Autodesk Inventor part; units mm, degrees
ref_plane "YZ Plane" through (0, 0, 0) normal (1, 0, 0) x (0, 1, 0)
ref_plane "XZ Plane" through (0, 0, 0) normal (0, 1, 0) x (-1, 0, 0)
ref_plane "XY Plane" through (0, 0, 0) normal (0, 0, 1) x (1, 0, 0)
sketch "Sketch1" plane through (0, 0, 0) normal (0, 1, 0) x (-1, 0, 0)
  line L0 (50, 0) -> (50, 40)
  line L1 (50, 40) -> (0, 40)
  line L2 (0, 40) -> (0, 0)
  line L3 (0, 0) -> (10, 0)
  line L4 (10, 0) -> (10, 10)
  line L5 (10, 10) -> (10, 30)
  circle A0 centre (10, 30) radius 3.1
  circle A1 centre (10, 10) radius 3.1
  line L6 (45.5, 0) -> (45.5, 11.4783)
  line L7 (0, 0) -> (33.5, 0)
  line L8 (35.5, 0) -> (35.5, 18.6699)
  line L9 (50, 40) -> (45.5, 40)
  line L10 (45.5, 40) -> (45.5, 35.5)
  line L11 (45.5, 35.5) -> (45.5, 34.5217)
  line L12 (45.5, 23) -> (33, 23)
  arc A2 (45.5, 11.4783) -> (33, 40) centre (33, 23) ccw
  line L13 (0, 0) -> (33.5, 0)
  line L14 (35.5, 0) -> (45.5, 0)
  line L15 (33.5, 0) -> (33.5, 18.0251)
  line L16 (0, 0) -> (33.5, 0)
  line L17 (35.5, 0) -> (45.5, 0)
  line L18 (33, 23) -> (28, 23)
  line L19 (33, 23) -> (38, 23)
  arc A3 (35.5, 18.6699) -> (38, 23) centre (33, 23) ccw
  arc A4 (28, 23) -> (33.5, 18.0251) centre (33, 23) ccw
  dimension "d0" = 50
  dimension "d1" = 40
  dimension "d2" = 10
  dimension "d3" = 10
  dimension "d4" = 20
  dimension "d5" = 6.2
  dimension "d6" = 6.2
  dimension "d7" = 45.5
  dimension "d8" = 35.5
  dimension "d9" = 4.5
  dimension "d10" = 4.5
  dimension "d13" = 12.5
  dimension "d14" = 12.5
  dimension "d15" = 2
extrude "Extrusion1" add sketch "Sketch1" along normal blind 25.4 contours A2 L6 L14 L8 A3 L12 L18 A4 L15 L7 L3 L2 L1
sketch "Sketch2" plane through (-33, 0, 40) normal (0, 0, 1) x (1, 0, 0)
  line L0 (33, 0) -> (33, 8.2)
  line L1 (33, 0) -> (33, 25.4)
  line L2 (33, 8.2) -> (16.5, 8.2)
  line L3 (16.5, 8.2) -> (16.5, 17.2)
  line L4 (16.5, 17.2) -> (33, 17.2)
  line L5 (33, 17.2) -> (33, 8.2)
  dimension "d18" = 8.2
  dimension "d19" = 16.5
  dimension "d20" = 9
extrude "Extrusion2" cut sketch "Sketch2" against normal through all
sketch "Sketch5" plane through (-28, 0, 23) normal (0, 0, -1) x (-1, 0, 0)
  line L0 (5, 25.4) -> (-4.4638, 26.228)
  line L1 (5, 25.4) -> (14.5, 25.4) construction
  line L2 (-4.4638, 26.228) -> (-3.5923, 36.1899)
  line L3 (-3.5923, 36.1899) -> (15.3354, 34.534)
  line L4 (15.3354, 34.534) -> (12.7207, 4.6481)
  line L5 (12.7207, 4.6481) -> (-6.207, 6.3041)
  line L6 (-6.207, 6.3041) -> (-3.5923, 36.1899)
  line L7 (3.2569, 5.4761) -> (5.8716, 35.3619)
  point P0 (-28, 0)
  dimension "d25" = 9.5
  dimension "d26" = 175
  dimension "d27" = 10
  dimension "d28" = 19
  dimension "d29" = 30
  dimension "d30" = 90
  dimension "d31" = 19
revolve "Revolution1" cut sketch "Sketch5" angle 360 about axis through (-31.2569, 5.4761, 23) along (-0.0871557, 0.9961947, 0) contours L7 L5 L6 L0 | L0 L2 L3 L7
sketch "Sketch6" plane through (-33.5, 5.2799, 18.0251) normal (-0.0871557, 0.9961947, 0) x (0.9961947, 0.0871557, 0)
  arc A0 (-0.2388, 4.1928) -> (1.7536, 4.512) centre (2.2517, -4.9749) ccw
  circle A1 centre (2.2517, -4.9749) radius 9.5
  point P0 (32.9124, 18.0251)
extrude "Extrusion3" cut sketch "Sketch6" against normal blind 10
properties part number "suporte-eixo"
Model file for the job. Use its own axes, mm. A direction names the side the tool comes from. Coordinates: 2 decimals unless noted, no trailing zeros. Loops run counter-clockwise (first coordinate to the right, second up) from the corner with the lowest first, then second, coordinate; pieces in that order, holes last. Notation, with made-up numbers: (54, 57.5) - (59, 57.5) arc R18 cw to (59, 83.5) - close; hole circle Ø5 at (-23.75, -32). An arc over 180 degrees is marked (long way). Answer as a JSON object with one key per item and string values. Group by question number.
(1) Probe line 1 along Z through (x, y) = (-10, 20.5); line 2 along X through (y, z) = (11, 8); line 3 along X through (y, z) = (20, 30). List the from-to ranges inside material, lowest first.
(2) Cut at B-B (x = -10). Give the cut face in (y, z).
(3) Cut at A-A (z = 10). Give the cut face in (x, y), then the cut area to 3 significant figures.
(4) Tool access for faces 4 (the face through (-16.5, 13, 20)), 5 (the face through (-19, 25.4, 20)), 6 (the face through (-33.5, 13, 7)), 7 (the face through (-45.5, 13, 6)), 8 (the face through (-40, 13, 0)): list every direction of +Z, -Z, +X, -X, +Y, -Y with a clear straight run to the whole face (end or side of a thin tool).
(5) Cut at D-D (z = 30). Give the cut face in (x, y), then the cut area to 3 significant figures.
(6) Flat gauge pins, fed straight in: pin 1 (5.5 mm diameter, centred on x = -10, z = 30, fed in from -Y); pin 2 (3 mm diameter, centred on y = 14.5, z = 17.5, fed in from -X); pin 3 (7 mm diameter, centred on y = 17.5, z = 5.5, fed in from -X); pin 4 (2 mm diameter, centred on y = 9.5, z = 13, fed in from -X). Where does each tip first touch, or does it go through?
(7) Two-plate mould, pull along Z, no slides. Class faces 1 (the face through (-17, 13, 0)), 2 (the face through (-8, 17.2, 20)), 3 (the face through (-6.9, 21.2, 9.9)): released by +Z, released by -Z, zero draft, split by the parting line, or undercut.
(8) Cut at C-C (x = -5). Give the cut face in (y, z).
Geometry says:
{
 "1": {"line 1": "z = 0 to 6.9, 13.1 to 26.9, 33.1 to 40", "line 2": "x = -45.5 to -35.5, -33.5 to -16.5", "line 3": "x = -48.49 to -38.97, -26.08 to -13.1, -6.9 to 0"},
 "2": {"outline": "(0, 0) - (8.2, 0) - (8.2, 6.9) - (0, 6.9) - close; (0, 13.1) - (8.2, 13.1) - (8.2, 26.9) - (0, 26.9) - close; (0, 33.1) - (8.2, 33.1) - (8.2, 40) - (0, 40) - close; (17.2, 0) - (25.4, 0) - (25.4, 6.9) - (17.2, 6.9) - close; (17.2, 13.1) - (25.4, 13.1) - (25.4, 26.9) - (17.2, 26.9) - close; (17.2, 33.1) - (25.4, 33.1) - (25.4, 40) - (17.2, 40) - close"},
 "3": {"outline": "(-45.5, 0) - (-35.5, 0) - (-35.5, 25.4) - (-45.5, 25.4) - close; (-33.5, 0) - (-13.1, 0) - (-13.1, 8.2) - (-16.5, 8.2) - (-16.5, 17.2) - (-13.1, 17.2) - (-13.1, 25.4) - (-33.5, 25.4) - close; (-6.9, 0) - (0, 0) - (0, 8.2) - (-6.9, 8.2) - close; (-6.9, 17.2) - (0, 17.2) - (0, 25.4) - (-6.9, 25.4) - close", "area": "855 mm^2"},
 "4": {"face 4": "+Z, -Z, +X", "face 5": "+Z, -Z, +X, -X, +Y", "face 6": "-Z, +Y, -Y", "face 7": "-Z, -X, +Y, -Y", "face 8": "-Z, +X, -X, +Y, -Y"},
 "5": {"outline": "(-48.49, 0) - (-37.22, 0) - (-37.65, 4.92) - (-39.45, 25.4) - (-48.49, 25.4) - close; (-26.55, 25.4) - (-24.86, 6.04) - (-24.33, 0) - (-13.1, 0) - (-13.1, 8.2) - (-16.5, 8.2) - (-16.5, 17.2) - (-13.1, 17.2) - (-13.1, 25.4) - close; (-6.9, 0) - (0, 0) - (0, 8.2) - (-6.9, 8.2) - close; (-6.9, 17.2) - (0, 17.2) - (0, 25.4) - (-6.9, 25.4) - close", "area": "654 mm^2"},
 "6": {"pin 1": "passes through", "pin 2": "stops at x = -49.52", "pin 3": "stops at x = -45.5", "pin 4": "stops at x = -47.42"},
 "7": {"face 1": "released by -Z", "face 2": "zero draft", "face 3": "undercut"},
 "8": {"outline": "(0, 0) - (8.2, 0) - (8.2, 40) - (0, 40) - close; (17.2, 0) - (25.4, 0) - (25.4, 40) - (17.2, 40) - close"}
}
